Part print with two shaded views. Sizes in mm from the minimum x, y, z corner. A direction names the side the tool comes from. Coordinates: 2 decimals unless noted, no trailing zeros. Write each loop counter-clockwise with the first axis right and the second up, starting at its lowest first coordinate (ties: lowest second). Pieces come first, ordered by that corner, then holes. Notation, with made-up numbers: (-10, 16.25) - (8, 16.25) arc R32 ccw to (8, 49.25) - close; hole circle Ø4 at (82.5, -28.5). An arc over 180 degrees is marked (long way). Answer in a Markdown table with one row per item. Add a question column.
Q1. Band-saw the part on C-C (x = 12). List the corners of the cut face in (y, z), and give its area (3 significant figures).
Q2. Pin check, flat tips, straight feed: pin 1 (0.5 mm diameter, centred on x = 14.5, y = 0.5, fed in from +Z); pin 2 (2 mm diameter, centred on x = 20, y = 10, fed in from +Z); pin 3 (2 mm diameter, centred on x = 9, y = 8.5, fed in from +Z); pin 4 (2 mm diameter, centred on x = 9.5, z = 3.5, fed in from -Y). Stop position of each tip, or through.
Q3. Band-saw the part on D-D (x = 4.25). List the corners of the cut face in (y, z).
Q4. Two-plate mould, pull along X, no slides. Class the marked faces 1 and 2: +X half, -X half, draft (parallel to the pull), parting line (faces both ways), or undercut.
Q5. Band-saw the part on B-B (y = 10). List the corners of the cut face in (x, z), and give its area (3 significant figures).
Q6. 3-axis set-ups, long thin cutter, end or side, ignore diameter. For the marked faces 3, 4 and 5: which of +Z, -Z, +X, -X, +Y, -Y reach the whole face in a straight line?
Q7. Drill centre lines: line 1 along Y through (x, z) = (18.25, 4.2); line 2 along Y through (x, z) = (4, 0.85); line 3 along X through (y, z) = (11.5, 3.1). Where is each one in solid material? Low to high. Write a range as from..to.
Q8. Band-saw the part on A-A (z = 3.25). List the corners of the cut face in (x, y), and give its area (3 significant figures).
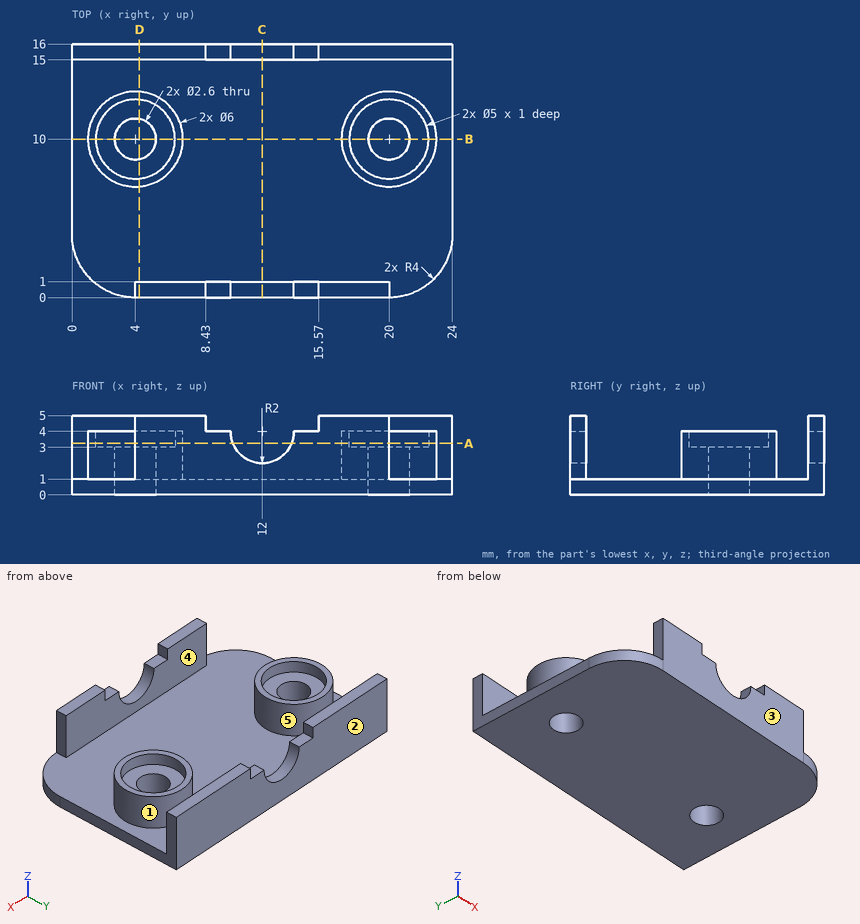
Checked values:
| question | item | result |
|---|---|---|
| 1 | outline | (0, 0) - (16, 0) - (16, 2) - (15, 2) - (15, 1) - (1, 1) - (1, 2) - (0, 2) - close |
| 1 | area | 18.0 mm² |
| 2 | pin 1 | stops at z = 4 |
| 2 | pin 2 | passes through |
| 2 | pin 3 | stops at z = 1 |
| 2 | pin 4 | stops at y = 0 |
| 3 | outline | (0, 0) - (8.72, 0) - (8.72, 3) - (7.51, 3) - (7.51, 4) - (7.01, 4) - (7.01, 1) - (1, 1) - (1, 5) - (0, 5) - close; (11.28, 0) - (16, 0) - (16, 5) - (15, 5) - (15, 1) - (12.99, 1) - (12.99, 4) - (12.49, 4) - (12.49, 3) - (11.28, 3) - close |
| 4 | face 1 | undercut |
| 4 | face 2 | draft |
| 5 | outline | (0, 0) - (2.7, 0) - (2.7, 3) - (1.5, 3) - (1.5, 4) - (1, 4) - (1, 1) - (0, 1) - close; (5.3, 0) - (18.7, 0) - (18.7, 3) - (17.5, 3) - (17.5, 4) - (17, 4) - (17, 1) - (7, 1) - (7, 4) - (6.5, 4) - (6.5, 3) - (5.3, 3) - close; (21.3, 0) - (24, 0) - (24, 1) - (23, 1) - (23, 4) - (22.5, 4) - (22.5, 3) - (21.3, 3) - close |
| 5 | area | 34.4 mm² |
| 6 | face 3 | +Z, -Z, +X, -X, -Y |
| 6 | face 4 | +Z, +X, -X |
| 6 | face 5 | +Z |
| 7 | line 1 | y = 0..1, 15..16 |
| 7 | line 2 | y = 0..8.7, 11.3..16 |
| 7 | line 3 | x = 1.4..2, 6..6.6, 17.4..18, 22..22.6 |
| 8 | outline | (0, 15) - (10.15, 15) - (10.15, 16) - (0, 16) - close; circle Ø6 at (4, 10); (4, 0) - (10.15, 0) - (10.15, 1) - (4, 1) - close; (13.85, 0) - (20, 0) - (20, 1) - (13.85, 1) - close; (13.85, 15) - (24, 15) - (24, 16) - (13.85, 16) - close; circle Ø6 at (20, 10); hole circle Ø5 at (4, 10); hole circle Ø5 at (20, 10) |
| 8 | area | 49.9 mm² |
